Source: CAD feature listing. Evaluate the final solid. Frame: model axes, mm. Face numbers are marked on the shaded views. A direction names the side the tool comes from. Coordinates: 2 decimals unless noted, no trailing zeros. Order: outer loops, then holes, each group sorted by start corner. A loop starts at its lowest first (then second) coordinate and runs counter-clockwise, first axis right, second up.
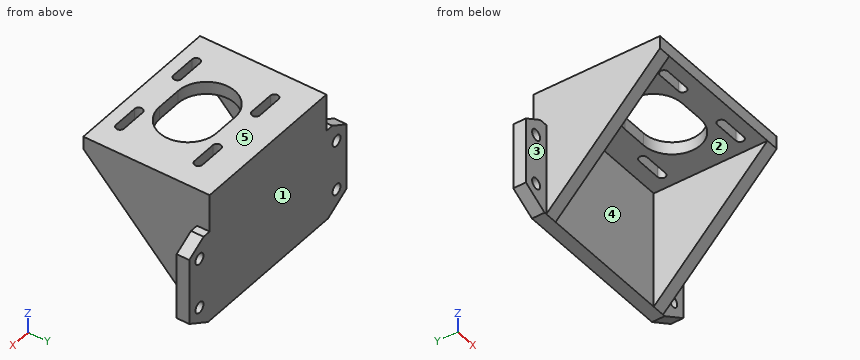
Autodesk Inventor part; units mm, degrees
ref_plane "XZ Plane" through (0, 0, 0) normal (0, 1, 0) x (-1, 0, 0)
ref_plane "XY Plane" through (0, 0, 0) normal (0, 0, 1) x (1, 0, 0)
ref_plane "Work Plane1" through (-118.9196, 128.4425, 80.2184) normal (0, -1, 0) x (0, 0, -1)
sketch "Sketch1" plane through (-118.9196, 128.4425, 80.2184) normal (0, -1, 0) x (0, 0, -1)
  line L0 (-4.2, -124) -> (-4.2, 744) construction
  line L1 (15.8, -124) -> (15.8, 744) construction
  line L2 (25.8, 100) -> (25.8, 520) construction
  line L3 (-21.85, -73.15) -> (24.8, -73.15)
  line L4 (24.8, -73.15) -> (24.8, 11.85)
  line L5 (24.8, 11.85) -> (-21.85, 11.85)
  line L6 (-21.85, 11.85) -> (-21.85, -73.15)
  line L7 (25.8, -30.65) -> (5.6685, -30.65) construction
  circle A0 centre (15.8, -67.65) radius 5.5 construction
  circle A1 centre (15.8, 6.35) radius 5.5 construction
  line L8 (5.8, -58.8473) -> (5.8, 42.3952) construction
  circle A2 centre (-4.2, -67.65) radius 5.5 construction
  circle A3 centre (-4.2, 6.35) radius 5.5 construction
  point P0 (80.2184, 118.9196)
  point P1 (18.9754, -73.15)
  point P2 (24.8, -26.5615)
  dimension "d0" = 1
  dimension "d1" = 47.65
  dimension "d3" = 11
  dimension "d4" = 63
  dimension "d7" = 0
  dimension "d9" = 10
  dimension "d10" = 10
extrude "Extrusion1" add sketch "Sketch1" along normal blind 5
ref_plane "Work Plane2" through (-149.5696, 123.4425, 102.0684) normal (1, 0, 0) x (0, 1, 0)
sketch "Sketch4" plane through (-192.0696, 128.4425, 102.0684) normal (0, 0, 1) x (1, 0, 0)
  line L0 (85, 0) -> (0, 0) construction
  line L1 (0, 0) -> (0, -5) construction
  line L2 (85, -5) -> (0, -5) construction
  line L3 (85, 0) -> (85, -5) construction
  line L4 (0, 0) -> (85, 0) construction
  line L5 (42.5, 0) -> (42.5, -58.6666) construction
  line L6 (11, 0) -> (74, 0)
  line L7 (74, 0) -> (74, -50)
  line L8 (74, -50) -> (11, -50)
  line L9 (11, -50) -> (11, 0)
  line L10 (27, -43.5) -> (58, -43.5) construction
  line L11 (58, -43.5) -> (58, -12.5) construction
  line L12 (58, -12.5) -> (27, -12.5) construction
  line L13 (27, -12.5) -> (27, -43.5) construction
  line L14 (27, -43.5) -> (58, -12.5) construction
  line L15 (58, -43.5) -> (27, -12.5) construction
  line L16 (32, -12.5) -> (22, -12.5) construction
  line L17 (32, -10.9) -> (22, -10.9)
  line L18 (22, -14.1) -> (32, -14.1)
  arc A0 (32, -14.1) -> (32, -10.9) centre (32, -12.5) ccw
  arc A1 (22, -10.9) -> (22, -14.1) centre (22, -12.5) ccw
  line L19 (53, -12.5) -> (63, -12.5) construction
  line L20 (53, -14.1) -> (63, -14.1)
  line L21 (63, -10.9) -> (53, -10.9)
  arc A2 (53, -10.9) -> (53, -14.1) centre (53, -12.5) ccw
  arc A3 (63, -14.1) -> (63, -10.9) centre (63, -12.5) ccw
  line L22 (32, -43.5) -> (22, -43.5) construction
  line L23 (32, -45.1) -> (22, -45.1)
  line L24 (22, -41.9) -> (32, -41.9)
  arc A4 (32, -45.1) -> (32, -41.9) centre (32, -43.5) ccw
  arc A5 (22, -41.9) -> (22, -45.1) centre (22, -43.5) ccw
  line L25 (53, -43.5) -> (63, -43.5) construction
  line L26 (53, -45.1) -> (63, -45.1)
  line L27 (63, -41.9) -> (53, -41.9)
  arc A6 (53, -41.9) -> (53, -45.1) centre (53, -43.5) ccw
  arc A7 (63, -45.1) -> (63, -41.9) centre (63, -43.5) ccw
  line L28 (37.5, -28) -> (47.5, -28) construction
  line L29 (37.5, -39.25) -> (47.5, -39.25)
  line L30 (47.5, -16.75) -> (37.5, -16.75)
  arc A8 (37.5, -16.75) -> (37.5, -39.25) centre (37.5, -28) ccw
  arc A9 (47.5, -39.25) -> (47.5, -16.75) centre (47.5, -28) ccw
  point P0 (192.0696, -128.4425)
  point P1 (42.5, -28)
  dimension "d14" = 63
  dimension "d15" = 45
  dimension "d16" = 31
  dimension "d17" = 31
  dimension "d18" = 3.2
  dimension "d19" = 10
  dimension "d21" = 10
  dimension "d22" = 1.6
  dimension "d23" = 10
  dimension "d24" = 10
  dimension "d25" = 1.6
  dimension "d26" = 1.6
  dimension "d27" = 22.5
  dimension "d28" = 10
extrude "Extrusion2" add sketch "Sketch4" along normal blind 5
sketch "Sketch5" plane through (-181.0696, 78.4425, 102.0684) normal (-1, 0, 0) x (0, 0, 1)
  line L0 (0, 45) -> (0, 0)
  line L1 (0, 45) -> (-46.65, 45)
  line L2 (-46.65, 50) -> (-46.65, 45)
  line L3 (0, 0) -> (0, 45)
  line L4 (-46.65, 45) -> (0, 0)
  point P0 (-102.0684, -78.4425)
extrude "Extrusion3" add sketch "Sketch5" against normal blind 5
sketch "Sketch6" plane through (-118.0696, 78.4425, 102.0684) normal (1, 0, 0) x (0, 0, -1)
  line L0 (0, 0) -> (46.65, 45)
  line L1 (0, 45) -> (46.65, 45)
  line L2 (0, 0) -> (0, 45)
  point P0 (102.0684, -78.4425)
extrude "Extrusion4" add sketch "Sketch6" against normal blind 5
sketch "Sketch7" plane through (-118.9196, 123.4425, 80.2184) normal (0, -1, 0) x (1, 0, 0)
  circle A0 centre (-67.65, -15.8) radius 5.5 construction
  circle A1 centre (-67.65, 4.2) radius 5.5 construction
  circle A2 centre (6.35, 4.2) radius 5.5 construction
  circle A3 centre (6.35, -15.8) radius 5.5 construction
  point P0 (118.9196, -80.2184)
hole "Hole1" at (-186.5696, 123.4425, 84.4184) at (-186.5696, 123.4425, 64.4184) at (-112.5696, 123.4425, 64.4184) at (-112.5696, 123.4425, 84.4184) direction (0, 1, 0) diameter 4.3 end through all
sketch "Sketch8" plane through (-118.9196, 123.4425, 80.2184) normal (0, -1, 0) x (1, 0, 0)
  circle A0 centre (-67.65, 4.2) radius 2.15
  circle A1 centre (-67.65, -15.8) radius 2.15
  line L0 (-62.15, -24.8) -> (-62.15, 21.85)
  line L1 (-62.15, 21.85) -> (-73.15, 21.85)
  line L2 (-73.15, 21.85) -> (-73.15, -24.8)
  line L3 (-73.15, -24.8) -> (-62.15, -24.8)
  circle A2 centre (6.35, -15.8) radius 2.15
  circle A3 centre (6.35, 4.2) radius 2.15
  line L4 (0.85, 21.85) -> (0.85, -24.8)
  line L5 (0.85, -24.8) -> (11.85, -24.8)
  line L6 (11.85, -24.8) -> (11.85, 21.85)
  line L7 (11.85, 21.85) -> (0.85, 21.85)
  line L8 (-73.15, 7.3754) -> (-65.3998, 11.85)
  line L9 (-73.15, -18.9754) -> (-62.15, -25.3263)
  line L10 (11.85, 7.3754) -> (4.0998, 11.85)
  line L11 (11.85, -18.9754) -> (0.85, -25.3263)
  line L12 (-65.3998, 11.85) -> (-62.15, 11.85)
  line L13 (4.0998, 11.85) -> (0.85, 11.85)
  point P0 (118.9196, -80.2184)
  point P1 (37.3678, 12.85)
  point P2 (-28.6678, 12.85)
  point P3 (1.7615, -24.8)
  point P4 (-63.0615, -24.8)
  point P5 (37.3678, 12.85)
  dimension "d42" = 60
  dimension "d43" = 5.5
  dimension "d44" = 60
  dimension "d45" = 5.5
  dimension "d46" = 60
  dimension "d47" = 5.5
  dimension "d48" = 60
  dimension "d49" = 5.5
  dimension "d53" = 7.65
  dimension "d54" = 7.65
extrude "Extrusion5" cut sketch "Sketch8" against normal blind 5 contours L12 L8 L2 L1 L0 | L3 L2 L9 | L7 L6 L10 L13 L4 | L11 L6 L5
equation "\"d1\" = MOTOR_HEIGHT"
equation "\"d9\" = d10"
equation "\"d19\" = SLOT_PLAY"
equation "\"d21\" = d19"
equation "\"d22\" = 0.5 * d18"
equation "\"d23\" = d19"
equation "\"d24\" = d19"
equation "\"d25\" = d22"
equation "\"d26\" = d22"
equation "\"d28\" = SLOT_PLAY"
equation "\"d44\" = d42"
equation "\"d45\" = d43"
equation "\"d47\" = d43"
equation "\"d49\" = d45"
equation "\"d54\" = d53"
equation "\"MOTOR_HEIGHT\" = 47.65"
equation "\"SLOT_PLAY\" = 10"
properties part number "MotorBracketV2"
1. Section query D-D on x = -164. Return loops of the section in (y, z), plus the area to 3 significant figures.
Findings:
outline: (78.44, 102.07) - (83.34, 102.07) - (83.34, 107.07) - (78.44, 107.07) - close; (86.54, 102.07) - (94.31, 102.07) - (94.31, 107.07) - (86.54, 107.07) - close; (106.58, 102.07) - (114.34, 102.07) - (114.34, 107.07) - (106.58, 107.07) - close; (117.54, 102.07) - (123.44, 102.07) - (123.44, 55.42) - (128.44, 55.42) - (128.44, 107.07) - (117.54, 107.07) - close
area: 390 mm2
2. Ray query, line 1 (X direction, y = 115, z = 72); line 2 (Z direction, x = -130, y = 120.5); line 3 (Y direction, x = -117, z = 84). Return the intervals inside material, ascending.
Findings:
line 1: x = -181.07 to -176.07, -123.07 to -118.07
line 2: z = 102.07 to 107.07
line 3: y = 123.44 to 128.44
3. Section query C-C on y = 103.5. Return loops of the section in (x, z).
Findings:
outline: (-181.07, 76.09) - (-176.07, 76.09) - (-176.07, 102.07) - (-165.4, 102.07) - (-165.4, 107.07) - (-181.07, 107.07) - close; (-133.74, 102.07) - (-123.07, 102.07) - (-123.07, 76.09) - (-118.07, 76.09) - (-118.07, 107.07) - (-133.74, 107.07) - close
4. Section query A-A on x = -151.5. Return loops of the section in (y, z), plus the area to 3 significant figures.
Findings:
outline: (78.44, 102.07) - (89.19, 102.07) - (89.19, 107.07) - (78.44, 107.07) - close; (111.69, 102.07) - (123.44, 102.07) - (123.44, 55.42) - (128.44, 55.42) - (128.44, 107.07) - (111.69, 107.07) - close
area: 371 mm2
5. Draft query along X for the marked faces 4 and 5. Return one class per face: released by +X, released by -X, zero draft, split by the parting line, or undercut.
Findings:
face 4: undercut
face 5: zero draft
6. Pin query (flat end, axial travel): P1, Ø9, axis at x = -188, z = 67.5, coming from the -Y side; P2, Ø4, axis at x = -186.57, z = 84.42, coming from the +Y side; P3, Ø22.5, axis at y = 109.5, z = 77.5, coming from the +X side; P4, Ø5, axis at x = -129, y = 93.5, coming from the -Z side. Return the tip coordinate at first contact, or that it passes through.
Findings:
P1: stops at y = 123.44
P2: passes through
P3: stops at x = -118.07
P4: stops at z = 102.07
7. Access query for the marked faces 1, 2 and 3. Directions: +Z, -Z, +X, -X, +Y, -Y. A direction counts if a zero-diameter tool reaches every point of the face in a straight line with its end or side. Return the directions, or none.
Findings:
face 1: +Z, -Z, +X, -X, +Y
face 2: -Z, -Y
face 3: +Z, -Z, -X, -Y
8. Section query B-B on z = 65. Return loops of the section in (x, y), plus the area to 3 significant figures.
Findings:
outline: (-192.07, 123.44) - (-188.64, 123.44) - (-188.64, 128.44) - (-192.07, 128.44) - close; (-184.5, 123.44) - (-181.07, 123.44) - (-181.07, 114.2) - (-176.07, 114.2) - (-176.07, 123.44) - (-123.07, 123.44) - (-123.07, 114.2) - (-118.07, 114.2) - (-118.07, 123.44) - (-114.64, 123.44) - (-114.64, 128.44) - (-184.5, 128.44) - close; (-110.5, 123.44) - (-107.07, 123.44) - (-107.07, 128.44) - (-110.5, 128.44) - close
area: 476 mm2
